Check sheet for the modelled part. Datum: model origin and axes. Units: mm. Round coordinates to 2 decimals unless told otherwise and drop trailing zeros. Order: outer loops, then holes, each group sorted by start corner. A loop starts at its lowest first (then second) coordinate and runs counter-clockwise, first axis right, second up. Notation, with made-up numbers: (-8.75, 28.25) -> (49.25, 28.25) arc R25 ccw to (49.25, 64.25) -> close; hole circle Ø2 at (-14.5, -29). An arc over 180 degrees is marked (long way). Answer in a Markdown table with one row per item.
from build123d import *

# Parameters (mm, degrees)
BOSS_EXTRUDE1_DEPTH = 6.223


with BuildPart() as part:
    # Sketch1 → Boss-Extrude1 (new body)
    with BuildSketch(Plane.XY):
        with BuildLine():
            Line((0, 15.9385), (0, 0))
            Line((0, 0), (30.504432116, 0))
            ThreePointArc((30.504432116, 0), (25.4, 19.05), (30.504432116, 38.1))
            Line((30.504432116, 38.1), (0, 38.1))
            Line((0, 38.1), (0, 22.1615))
            ThreePointArc((0, 22.1615), (2.20016275, 21.25016275), (3.1115, 19.05))
            ThreePointArc((3.1115, 19.05), (2.20016275, 16.84983725), (0, 15.9385))
        make_face()
        with BuildLine():
            Line((30.504432116, 0), (0, 0))
            Line((0, 0), (0, 15.9385))
            ThreePointArc((0, 15.9385), (-3.1115, 19.05), (0, 22.1615))
            Line((0, 22.1615), (0, 38.1))
            Line((0, 38.1), (30.504432116, 38.1))
            ThreePointArc((30.504432116, 38.1), (31.111611101, 39.114951146), (31.75, 40.110567419))
            ThreePointArc((31.75, 40.110567419), (-38.1, 19.05), (31.75, -2.010567419))
            ThreePointArc((31.75, -2.010567419), (31.111611101, -1.014951146), (30.504432116, 0))
        make_face()
        with BuildLine():
            ThreePointArc((31.75, 40.110567419), (31.111611101, 39.114951146), (30.504432116, 38.1))
            Line((30.504432116, 38.1), (32.995567884, 38.1))
            ThreePointArc((32.995567884, 38.1), (32.388388899, 39.114951146), (31.75, 40.110567419))
        make_face()
        with BuildLine():
            Line((63.5, 0), (32.995567884, 0))
            ThreePointArc((32.995567884, 0), (32.388388899, -1.014951146), (31.75, -2.010567419))
            ThreePointArc((31.75, -2.010567419), (74.498522628, -17.427972806), (101.6, 19.05))
            ThreePointArc((101.6, 19.05), (74.498522628, 55.527972806), (31.75, 40.110567419))
            ThreePointArc((31.75, 40.110567419), (32.388388899, 39.114951146), (32.995567884, 38.1))
            Line((32.995567884, 38.1), (63.5, 38.1))
            Line((63.5, 38.1), (63.5, 22.1615))
            ThreePointArc((63.5, 22.1615), (65.70016275, 21.25016275), (66.6115, 19.05))
            ThreePointArc((66.6115, 19.05), (65.70016275, 16.84983725), (63.5, 15.9385))
            Line((63.5, 15.9385), (63.5, 0))
        make_face()
        with BuildLine():
            ThreePointArc((30.504432116, 38.1), (25.4, 19.05), (30.504432116, 0))
            Line((30.504432116, 0), (32.995567884, 0))
            ThreePointArc((32.995567884, 0), (36.801773982, 9.188994382), (38.1, 19.05))
            ThreePointArc((38.1, 19.05), (36.801773982, 28.911005618), (32.995567884, 38.1))
            Line((32.995567884, 38.1), (30.504432116, 38.1))
        make_face()
        with BuildLine():
            ThreePointArc((38.1, 19.05), (36.801773982, 9.188994382), (32.995567884, 0))
            Line((32.995567884, 0), (63.5, 0))
            Line((63.5, 0), (63.5, 15.9385))
            ThreePointArc((63.5, 15.9385), (60.3885, 19.05), (63.5, 22.1615))
            Line((63.5, 22.1615), (63.5, 38.1))
            Line((63.5, 38.1), (32.995567884, 38.1))
            ThreePointArc((32.995567884, 38.1), (36.801773982, 28.911005618), (38.1, 19.05))
        make_face()
        with BuildLine():
            Line((32.995567884, 0), (30.504432116, 0))
            ThreePointArc((30.504432116, 0), (31.111611101, -1.014951146), (31.75, -2.010567419))
            ThreePointArc((31.75, -2.010567419), (32.388388899, -1.014951146), (32.995567884, 0))
        make_face()
    extrude(amount=BOSS_EXTRUDE1_DEPTH)


solid = part.part
Item 1: Mould release check, pull along X, two halves, no side actions. Record for faces 1 (the flat face through (31, 20, 6.223)), 2 (the cylindrical face through (-38.076, 20.413, 3.068)): pulls with the +X half, pulls with the -X half, needs draft (parallel to the pull), parting line crosses it, or undercut.
Result sheet:
| item | result |
|---|---|
| face 1 | needs draft |
| face 2 | undercut |
Item 2: Depth check by flat-ended pin: P1, Ø1.5, axis at x = -19.5, z = 2.5, coming from the +Y side; P2, Ø3, axis at y = -4, z = 3, coming from the -X side; P3, Ø1.5, axis at y = 25, z = 3.5, coming from the +X side. Enter the tip coordinate at first touch or a pass-through.
Result sheet:
| item | result |
|---|---|
| P1 | stops at y = 52.22 |
| P2 | stops at x = -31.42 |
| P3 | stops at x = 101.24 |
Item 3: Cross-section at C-C (y = 51). Record the boundary of the cut face in (x, z), and give its area (3 significant figures).
Result sheet:
| item | result |
|---|---|
| outline | (-20.76, 0) -> (20.76, 0) -> (20.76, 6.22) -> (-20.76, 6.22) -> close; (42.74, 0) -> (84.26, 0) -> (84.26, 6.22) -> (42.74, 6.22) -> close |
| area | 517 mm^2 |
Item 4: Cross-section at D-D (x = -14). Record the boundary of the cut face in (y, z).
Result sheet:
| item | result |
|---|---|
| outline | (-16.38, 0) -> (54.48, 0) -> (54.48, 6.22) -> (-16.38, 6.22) -> close |
Item 5: Cross-section at A-A (y = 42). Record the boundary of the cut face in (x, z), and give its area (3 significant figures).
Result sheet:
| item | result |
|---|---|
| outline | (-30.41, 0) -> (30.41, 0) -> (30.41, 6.22) -> (-30.41, 6.22) -> close; (33.09, 0) -> (93.91, 0) -> (93.91, 6.22) -> (33.09, 6.22) -> close |
| area | 757 mm^2 |
Item 6: Cross-section at B-B (z = 4). Record the boundary of the cut face in (x, y).
Result sheet:
| item | result |
|---|---|
| outline | (31.75, -2.01) arc R38.1 ccw (long way) to (31.75, 40.11) arc R38.1 ccw (long way) to start; hole circle Ø6.22 at (0, 19.05); hole circle Ø6.22 at (63.5, 19.05) |
Item 7: Scan lines: line 1 (X direction, y = 53, z = 2.5); line 2 (X direction, y = 43, z = 3.5); line 3 (Y direction, x = 91, z = 1.5). Record each from-to range of solid material in increasing order. Write a range as [from, to].
Result sheet:
| item | result |
|---|---|
| line 1 | x = [-17.29, 17.29], [46.21, 80.79] |
| line 2 | x = [-29.63, 29.63], [33.87, 93.13] |
| line 3 | y = [-7.32, 45.42] |
